Check sheet for the modelled part. Datum: model origin and axes. Units: mm. A direction names the side the tool comes from. Coordinates: 2 decimals unless noted, no trailing zeros. Write each loop counter-clockwise with the first axis right and the second up, starting at its lowest first coordinate (ties: lowest second). Pieces come first, ordered by that corner, then holes. Notation, with made-up numbers: (35.5, 15) - (69.5, 15) arc R28 ccw to (69.5, 46) - close; hole circle Ø2 at (-36.75, 37). An arc over 180 degrees is marked (long way). Write each question's results on one line, items separated by ' | '.
from build123d import *

# Parameters (mm, degrees)
ESQUISSE1_R        = 2.25
BOSS_EXTRU_1_DEPTH = 4
CONG_2_R           = 6
CONG_3_R           = 20
ESQUISSE2_R        = 10.75
BOSS_EXTRU_2_DEPTH = 4.5


with BuildPart() as part:
    # Esquisse1 → Boss.-Extru.1 (new body)
    with BuildSketch(Plane.XY):
        Polygon((-55, 20), (-27.5, 0), (0, 20), (0, 40), (-55, 40), align=None)
        with Locations((-47.5, 32.5)):
            Circle(ESQUISSE1_R, mode=Mode.SUBTRACT)
        with Locations((-7.5, 32.5)):
            Circle(ESQUISSE1_R, mode=Mode.SUBTRACT)
        with Locations((-27.5, 7.5)):
            Circle(ESQUISSE1_R, mode=Mode.SUBTRACT)
    extrude(amount=BOSS_EXTRU_1_DEPTH)

    # Congé2
    cong_2_edges = [part.edges().sort_by_distance(p)[0] for p in [
        (-55, 40, 2),
        (0, 40, 2),
        (-27.5, 0, 2),
    ]]
    fillet(cong_2_edges, radius=CONG_2_R)

    # Congé3
    cong_3_edges = [part.edges().sort_by_distance(p)[0] for p in [
        (0, 20, 2),
        (-55, 20, 2),
    ]]
    fillet(cong_3_edges, radius=CONG_3_R)

    # Esquisse2 → Boss.-Extru.2 (add)
    with BuildSketch(Plane(origin=(0, 0, 0), x_dir=(-1, 0, 0), z_dir=(0, 0, -1))):
        with Locations(Location((27.5, 27.5, 0), (0, 0, 180))):  # turned: the seam where the file's is
            Circle(ESQUISSE2_R)
    extrude(amount=BOSS_EXTRU_2_DEPTH)

    # Esquisse3 → Enlèvement de matière-Révolution5 (revolve, cut)
    with BuildSketch(Plane(origin=(0, 0, -4.5), x_dir=(-1, 0, 0), z_dir=(0, 0, -1))):
        with BuildLine():
            Line((27.5, 30.25), (27.5, 24.75))
            ThreePointArc((27.5, 24.75), (24.75, 27.5), (27.5, 30.25))
        make_face()
    revolve(axis=Axis((-27.5, 30.25, -4.5), (0, -1, 0)), mode=Mode.SUBTRACT)


solid = part.part
1. Go/stop test with flat-tipped pins: pin 1 (8 mm diameter, centred on x = -9, y = 13, fed in from -Z); pin 2 (2 mm diameter, centred on y = 15.5, z = -2, fed in from +X). Record where each tip stops, or that it passes through.
Values follow:
pin 1: stops at z = 0 | pin 2: passes through
2. Draft check along Y on faces 3 (the cylindrical face through (-1.804, 38.289, 2.028)), 4 (the cylindrical face through (-52.76, 20.99, 2.03)), 5 (the flat face through (0, 32, 2)), 6 (the cylindrical face through (-7.79, 34.73, 1.97)). Enter one of: pulls with the +Y half, pulls with the -Y half, needs draft (parallel to the pull), parting line crosses it, or undercut.
Values follow:
face 3: pulls with the +Y half | face 4: pulls with the -Y half | face 5: needs draft | face 6: undercut
3. Access from +Z, -Z, +X, -X, +Y, -Y to the whole of each face (thin tool, end or side, straight path). Record for faces 1 (the cylindrical face through (-17.57, 31.62, -2.22)), 2 (the cylindrical face through (-53.289, 38.196, 2.028)).
Values follow:
face 1: -Z | face 2: +Z, -Z, -X, +Y
4. Sectioned sample at C-C (y = 32.5). Record the cut outline in (x, z), then the cut area to 3 significant figures.
Values follow:
outline: (-55, 0) - (-49.75, 0) - (-49.75, 4) - (-55, 4) - close; (-45.25, 0) - (-37.02, 0) - (-37.02, -4.5) - (-17.98, -4.5) - (-17.98, 0) - (-9.75, 0) - (-9.75, 4) - (-45.25, 4) - close; (-5.25, 0) - (0, 0) - (0, 4) - (-5.25, 4) - close | area: 270 mm^2
5. Sectioned sample at A-A (x = -48). Record the cut outline in (y, z).
Values follow:
outline: (14.99, 0) - (30.31, 0) - (30.31, 4) - (14.99, 4) - close; (34.69, 0) - (40, 0) - (40, 4) - (34.69, 4) - close
6. Sectioned sample at B-B (z = 3.25). Record the cut outline in (x, y).
Values follow:
outline: (-55, 30.18) arc R20 ccw to (-46.76, 14.01) - (-31.03, 2.57) arc R6 ccw to (-23.97, 2.57) - (-8.24, 14.01) arc R20 ccw to (0, 30.18) - (0, 34) arc R6 ccw to (-6, 40) - (-49, 40) arc R6 ccw to (-55, 34) - close; hole circle Ø4.5 at (-47.5, 32.5); hole circle Ø4.5 at (-27.5, 7.5); hole circle Ø4.5 at (-7.5, 32.5)
7. Sectioned sample at D-D (y = 27.5). Record the cut outline in (x, z).
Values follow:
outline: (-54.82, 0) - (-38.25, 0) - (-38.25, -4.5) - (-30.25, -4.5) arc R2.75 cw to (-24.75, -4.5) - (-16.75, -4.5) - (-16.75, 0) - (-0.18, 0) - (-0.18, 4) - (-54.82, 4) - close
8. Material ranges on L1, parallel to Y at x = -27.5, z = 2.25; L2, parallel to Y at x = -47.5, z = 2.3; L3, parallel to Z at x = -10.5, y = 37.5, recorded low to high. Write a range as [from, to].
Values follow:
L1: y = [1.42, 5.25], [9.75, 40] | L2: y = [14.57, 30.25], [34.75, 40] | L3: z = [0, 4]
